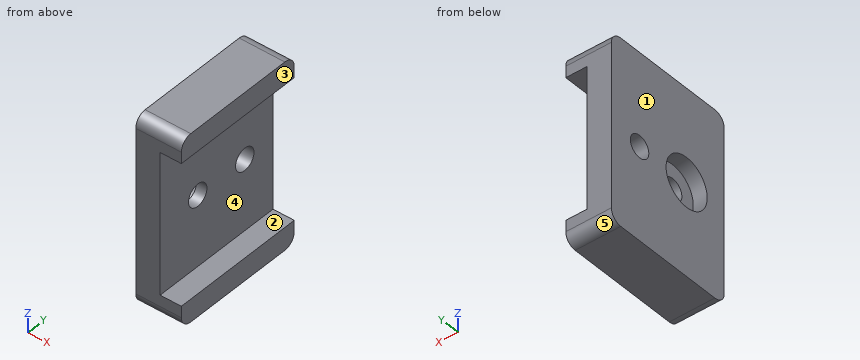
from build123d import *

# Parameters (mm, degrees)
BOSS_EXTRUDE1_DEPTH                                 = 5.461
F_10_CLEARANCE_HOLE1_D                              = 4.9784
CBORE_FOR_10_BINDING_HEAD_MACHINE_SCREW_D           = 4.9784
CBORE_FOR_10_BINDING_HEAD_MACHINE_SCREW_CBORE_D     = 11.1125
CBORE_FOR_10_BINDING_HEAD_MACHINE_SCREW_CBORE_DEPTH = 3.1242
SKETCH10_W                                          = 5.08
SKETCH10_H                                          = 30.48
BOSS_EXTRUDE2_DEPTH                                 = 4.7625
FILLET2_R                                           = 2.54


with BuildPart() as part:
    # Sketch1 → Boss-Extrude1 (new body)
    with BuildSketch(Plane(origin=(0, 0, 0), x_dir=(0, 0, -1), z_dir=(1, 0, 0))):
        Polygon((-15.875, -15.24), (15.875, -15.24), (20.955, -15.24), (20.955, 15.24), (15.875, 15.24), (-15.875, 15.24), (-20.955, 15.24), (-20.955, -15.24), align=None)
    extrude(amount=BOSS_EXTRUDE1_DEPTH)

    # #10 Clearance Hole1 (through all)
    with Locations(Plane.ZY):
        with Locations((0, 7.62)):
            Hole(F_10_CLEARANCE_HOLE1_D / 2)

    # CBORE for #10 Binding Head Machine Screw1 (through all)
    with Locations(Plane.ZY):
        with Locations((0, -5.08)):
            CounterBoreHole(CBORE_FOR_10_BINDING_HEAD_MACHINE_SCREW_D / 2, CBORE_FOR_10_BINDING_HEAD_MACHINE_SCREW_CBORE_D / 2, CBORE_FOR_10_BINDING_HEAD_MACHINE_SCREW_CBORE_DEPTH)

    # Sketch10 → Boss-Extrude2 (add)
    with BuildSketch(Plane(origin=(5.461, 0, 0), x_dir=(0, 0, -1), z_dir=(1, 0, 0))):
        with Locations((-18.415, 0)):
            Rectangle(SKETCH10_W, SKETCH10_H)
        with Locations((18.415, 0)):
            Rectangle(SKETCH10_W, SKETCH10_H)
    extrude(amount=BOSS_EXTRUDE2_DEPTH)

    # Fillet2
    fillet2_edges = [part.edges().sort_by_distance(p)[0] for p in [
        (5.11175, 15.24, -20.955),
        (5.11175, -15.24, -20.955),
        (5.11175, -15.24, 20.955),
        (5.11175, 15.24, 20.955),
    ]]
    fillet(fillet2_edges, radius=FILLET2_R)


solid = part.part
Here's how the part is built. I have some questions about the finished solid (model axes, mm). Face numbers are marked on the shaded views. A direction names the side the tool comes from. Coordinates: 2 decimals unless noted, no trailing zeros. Write each loop counter-clockwise with the first axis right and the second up, starting at its lowest first coordinate (ties: lowest second). Pieces come first, ordered by that corner, then holes.
Item 1: I want a section at D-D on x = 7.5. Write out the boundary of the cut face in (y, z) (3 decimals), and give its area (3 significant figures).
Item 2: If we mould it in two halves opening along Z, with no side actions, what happens to the marked faces 3, 4 and 5? For each: +Z half, -Z half, draft (parallel to the pull), parting line (faces both ways), or undercut.
Item 3: I want a section at B-B on z = 0. Write out the boundary of the cut face in (x, y), and give its area (3 significant figures).
Item 4: If I drill on line 1 (Y direction, x = 1.2, z = 0); line 2 (Y direction, x = 4, z = 0); line 3 (Z direction, x = 9.25, y = 0) (3 decimals), over which ranges is the centre line in solid material (lowest first)?
Item 5: Will this pin go through, and if not, where does the flat tip stop? pin 1 (15 mm diameter, centred on y = 5.5, z = -4.5, fed in from +X).
Item 6: On a 3-axis mill with a long thin cutter (end or side, diameter ignored), from which of +Z, -Z, +X, -X, +Y, -Y can I reach the whole of each face in a straight line? I mean the marked faces 1 and 2. Say none if no direction works.
Item 7: I want a section at C-C on y = -5.08. Write out the boundary of the cut face in (x, z) (1 decimal).
Item 8: I want a section at A-A on x = 1.5. Write out the boundary of the cut face in (y, z) (1 decimal), and give its area (3 significant figures).
Findings below:
1. outline: (-15.24, -18.415) arc R2.54 ccw to (-12.7, -20.955) - (12.7, -20.955) arc R2.54 ccw to (15.24, -18.415) - (15.24, -15.875) - (-15.24, -15.875) - close; (-15.24, 15.875) - (15.24, 15.875) - (15.24, 18.415) arc R2.54 ccw to (12.7, 20.955) - (-12.7, 20.955) arc R2.54 ccw to (-15.24, 18.415) - close
1. area: 304 mm2
2. face 3: draft
2. face 4: undercut
2. face 5: -Z half
3. outline: (0, -15.24) - (5.46, -15.24) - (5.46, -7.57) - (3.12, -7.57) - (3.12, -10.64) - (0, -10.64) - close; (0, 0.48) - (3.12, 0.48) - (3.12, -2.59) - (5.46, -2.59) - (5.46, 5.13) - (0, 5.13) - close; (0, 10.11) - (5.46, 10.11) - (5.46, 15.24) - (0, 15.24) - close
3. area: 92.9 mm2
4. line 1: y = -15.24 to -10.64, 0.48 to 5.13, 10.11 to 15.24
4. line 2: y = -15.24 to -7.57, -2.59 to 5.13, 10.11 to 15.24
4. line 3: z = -20.955 to -15.875, 15.875 to 20.955
5. pin 1: stops at x = 5.46
6. face 1: +Z, -Z, -X, +Y, -Y
6. face 2: +X, +Y, -Y
7. outline: (0, -21) - (10.2, -21) - (10.2, -15.9) - (5.5, -15.9) - (5.5, -2.5) - (3.1, -2.5) - (3.1, -5.6) - (0, -5.6) - close; (0, 5.6) - (3.1, 5.6) - (3.1, 2.5) - (5.5, 2.5) - (5.5, 15.9) - (10.2, 15.9) - (10.2, 21) - (0, 21) - close
8. outline: (-15.2, -18.4) arc R2.5 ccw to (-12.7, -21) - (12.7, -21) arc R2.5 ccw to (15.2, -18.4) - (15.2, 18.4) arc R2.5 ccw to (12.7, 21) - (-12.7, 21) arc R2.5 ccw to (-15.2, 18.4) - close; hole circle Ø11.1 at (-5.1, 0); hole circle Ø5 at (7.6, 0)
8. area: 1,160 mm2
